Geometry check sheet. Reference: drawing and pictorial views, mm from the part's lowest x, y, z. Give positions to 0.01 mm unless a question says otherwise; leave off trailing zeros. Loops run counter-clockwise (first coordinate to the right, second up) from the corner with the lowest first, then second, coordinate; pieces in that order, holes last. Notation, with made-up numbers: (79.25, 73.25) -> (91.25, 73.25) arc R20 cw to (91.25, 99.25) -> close; hole circle Ø6 at (-24, -0.5). An arc over 180 degrees is marked (long way). One line per item, written item: value. Start each with the question number.
(1) Sectioned sample at A-A, the plane z = 1.7. Record the cut outline in (x, y).
(2) Sectioned sample at B-B, the plane x = 25. Record the cut outline in (y, z).
(3) Scan lines: line 1 along X through (y, z) = (23, 4.5); line 2 along Y through (x, z) = (25.5, 4.35); line 3 along Y through (x, z) = (26.5, 3.3). Record each from-to range of solid material in increasing order. Write a range as from..to.
(4) Draft check along X on the marked faces 1, 2 and 3. Enter one of: pulls with the +X half, pulls with the -X half, needs draft (parallel to the pull), parting line crosses it, or undercut.
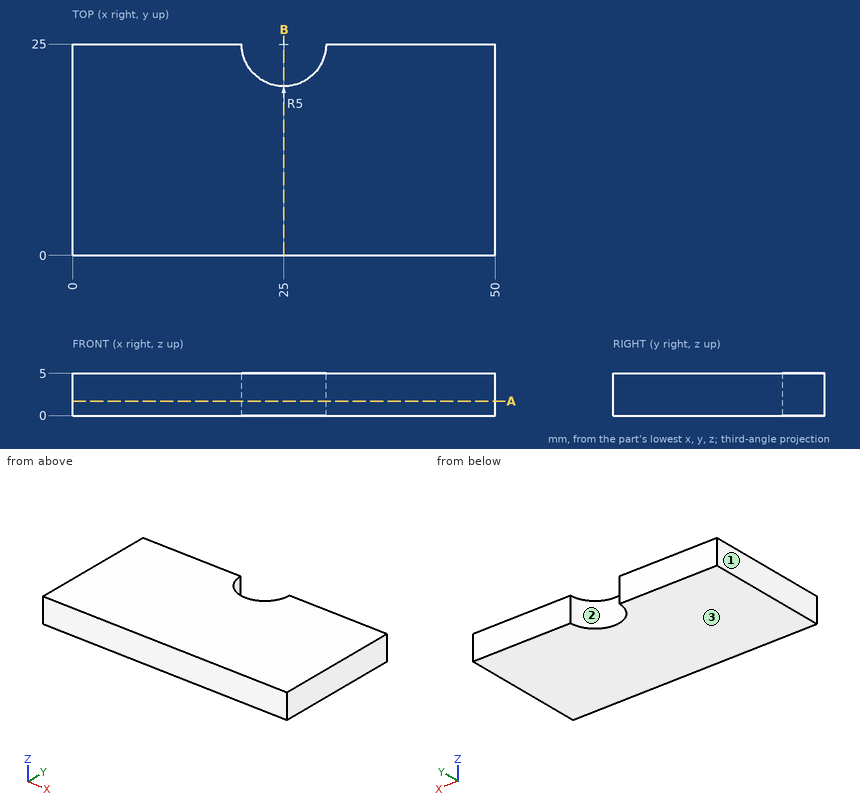
Calculated:
1. outline: (0, 0) -> (50, 0) -> (50, 25) -> (30, 25) arc R5 cw to (20, 25) -> (0, 25) -> close
2. outline: (0, 0) -> (20, 0) -> (20, 5) -> (0, 5) -> close
3. line 1: x = 0..20.42, 29.58..50
3. line 2: y = 0..20.03
3. line 3: y = 0..20.23
4. face 1: pulls with the -X half
4. face 2: undercut
4. face 3: needs draft
